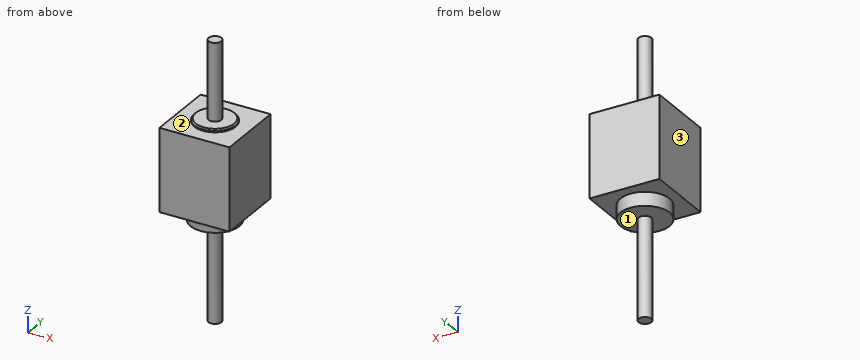
```python
from build123d import *

# Parameters (mm, degrees)
SKETCH1_W           = 2.54
SKETCH1_H           = 2.54
BOSS_EXTRUDE1_DEPTH = 3
SKETCH2_R           = 0.23
BOSS_EXTRUDE2_DEPTH = 4.1
SKETCH3_R           = 0.89
BOSS_EXTRUDE3_DEPTH = 0.5
SKETCH4_R           = 0.23
BOSS_EXTRUDE4_DEPTH = 2.9
SKETCH5_R           = 0.75
BOSS_EXTRUDE5_DEPTH = 0.1
CHAMFER1_SIZE       = 0.05


with BuildPart() as part:
    # Sketch1 → Boss-Extrude1 (new body)
    with BuildSketch(Plane.XY):
        Rectangle(SKETCH1_W, SKETCH1_H)
    extrude(amount=BOSS_EXTRUDE1_DEPTH)

    # Sketch2 → Boss-Extrude2 (add)
    with BuildSketch(Plane(origin=(0, 0, 0), x_dir=(-1, 0, 0), z_dir=(0, 0, -1))):
        Circle(SKETCH2_R)
    extrude(amount=BOSS_EXTRUDE2_DEPTH)

    # Sketch3 → Boss-Extrude3 (add)
    with BuildSketch(Plane(origin=(0, 0, 0), x_dir=(-1, 0, 0), z_dir=(0, 0, -1))):
        Circle(SKETCH3_R)
    extrude(amount=BOSS_EXTRUDE3_DEPTH)

    # Sketch4 → Boss-Extrude4 (add)
    with BuildSketch(Plane.XY.offset(3)):
        Circle(SKETCH4_R)
    extrude(amount=BOSS_EXTRUDE4_DEPTH)

    # Sketch5 → Boss-Extrude5 (add)
    with BuildSketch(Plane.XY.offset(3)):
        Circle(SKETCH5_R)
    extrude(amount=BOSS_EXTRUDE5_DEPTH)

    # Chamfer1
    chamfer1_edges = [part.edges().sort_by_distance(p)[0] for p in [
        (-0.75, 0, 3.1),
    ]]
    chamfer(chamfer1_edges, length=CHAMFER1_SIZE)


solid = part.part
```
Check sheet for the modelled part. Datum: model origin and axes. Units: mm. Face numbers are marked on the shaded views. A direction names the side the tool comes from. Coordinates: 2 decimals unless noted, no trailing zeros. Write each loop counter-clockwise with the first axis right and the second up, starting at its lowest first coordinate (ties: lowest second). Pieces come first, ordered by that corner, then holes. Notation, with made-up numbers: M 78,15.25 L 117,15.25 A26 ccw 117,41.25 Z; hole C 29.25,68.5 d8. An arc over 180 degrees is marked long. Use one line per item in the form item = value.
Item 1: Gauge pin test, flat end, axial feed: pin 1 Ø1.5 at (x, z) = (0, 4) entering from -Y. Record the tip position at first contact, or that the pin passes through.
Answer below:
pin_1 = -0.23
Item 2: Set-up check for the marked faces 1, 2 and 3: record each of +Z, -Z, +X, -X, +Y, -Y from which the full face is reachable in a straight line by a thin tool's end or side.
Answer below:
face_1 = -Z
face_2 = +Z
face_3 = +Z, -Z, -X, +Y, -Y
Item 3: Sectioned sample at C-C, the plane z = -3.5. Record the cut outline in (x, y), and give its area (3 significant figures).
Answer below:
outline = C 0,0 d0.46
area = 0.166 mm^2
Item 4: Sectioned sample at A-A, the plane x = 0. Record the cut outline in (y, z).
Answer below:
outline = M -1.27,0 L -0.89,0 L -0.89,-0.5 L -0.23,-0.5 L -0.23,-4.1 L 0.23,-4.1 L 0.23,-0.5 L 0.89,-0.5 L 0.89,0 L 1.27,0 L 1.27,3 L 0.75,3 L 0.75,3.05 L 0.7,3.1 L 0.23,3.1 L 0.23,5.9 L -0.23,5.9 L -0.23,3.1 L -0.7,3.1 L -0.75,3.05 L -0.75,3 L -1.27,3 Z
Item 5: Material ranges on L1, parallel to Z at x = 0.45, y = -0.1; L2, parallel to Y at x = 0, z = -2.75; L3, parallel to Z at x = -0.85, y = 0.35, recorded low to high. Write a range as from..to.
Answer below:
L1 = -0.5..3.1
L2 = -0.23..0.23
L3 = 0..3
